Autodesk Inventor part; units mm, degrees
sketch "Sketch_2" plane through (0, 0, 0) normal (0, 1, 0) x (-1, 0, 0)
  line L0 (14.6744, 3.8205) -> (14.6744, 4.3333)
  line L1 (14.6744, 4.3333) -> (13.0333, 4.3333)
  arc A0 (13.0333, 4.3333) -> (12.1103, 3.4103) centre (13.0333, 3.4103) ccw
  line L2 (12.1103, 3.4103) -> (12.1103, 1.4103)
  arc A1 (11.7, 1) -> (12.1103, 1.4103) centre (11.7, 1.4103) ccw
  line L3 (11.7, 1) -> (-0.3, 1)
  arc A2 (-0.7103, 1.4103) -> (-0.3, 1) centre (-0.3, 1.4103) ccw
  line L4 (-0.7103, 1.4103) -> (-0.7103, 3.4103)
  arc A3 (-0.7103, 3.4103) -> (-1.6333, 4.3333) centre (-1.6333, 3.4103) ccw
  line L5 (-1.6333, 4.3333) -> (-3.2744, 4.3333)
  line L6 (-3.2744, 4.3333) -> (-3.2744, 3.8205)
  line L7 (-3.2744, 3.8205) -> (-1.6333, 3.8205)
  arc A4 (-1.2231, 3.4103) -> (-1.6333, 3.8205) centre (-1.6333, 3.4103) ccw
  line L8 (-1.2231, 3.4103) -> (-1.2231, 1.4103)
  arc A5 (-1.2231, 1.4103) -> (-0.3, 0.4872) centre (-0.3, 1.4103) ccw
  line L9 (-0.3, 0.4872) -> (11.7, 0.4872)
  arc A6 (11.7, 0.4872) -> (12.6231, 1.4103) centre (11.7, 1.4103) ccw
  line L10 (12.6231, 1.4103) -> (12.6231, 3.4103)
  arc A7 (13.0333, 3.8205) -> (12.6231, 3.4103) centre (13.0333, 3.4103) ccw
  line L11 (13.0333, 3.8205) -> (14.6744, 3.8205)
  dimension "d13" = 12
extrude "Extrusion1" add sketch "Sketch_2" along normal blind 161
sketch "Sketch_6" plane through (0, 0, 0) normal (0, 0, 1) x (1, 0, 0)
  arc A0 (-8.7098, 4.8974) -> (-3.5098, 4.8974) centre (-6.1098, 4.8974) ccw
  line L0 (-3.5098, 4.8974) -> (-3.5098, 17.6974)
  arc A1 (-3.5098, 17.6974) -> (-8.7098, 17.6974) centre (-6.1098, 17.6974) ccw
  line L1 (-8.7098, 17.6974) -> (-8.7098, 4.8974)
extrude "Extrusion2" cut sketch "Sketch_6" along normal blind 1
pattern_linear "Rectangular Pattern1" count 80 spacing 23 along (0, 1, 0) of "Extrusion2"
properties part number "PP0735H(1)"
Source: CAD feature listing. Evaluate the final solid. Frame: model axes, mm. A direction names the side the tool comes from. Round coordinates to 2 decimals unless told otherwise and drop trailing zeros. Write each loop counter-clockwise with the first axis right and the second up, starting at its lowest first coordinate (ties: lowest second). Pieces come first, ordered by that corner, then holes. Notation, with made-up numbers: M -10,-21 L 16,-21 A22 cw 16,-10 Z; hole C 46.5,63.25 d3. An arc over 180 degrees is marked long. Use CSV: the item, a comma, the result in double quotes. Start each with the question number.
Q1. Cut plane A-A on z = 2.2. Output: boundary loops of the cut face in (x, y).
Q2. First-contact query: P1, Ø0.6, axis at y = 99.5, z = 3, coming from the +X side; P2, Ø0.6, axis at y = 125.5, z = 0.5, coming from the +X side; P3, Ø1.5, axis at y = 77, z = 1.5, coming from the -X side. Flat tips, straight axial feed; report the tip coordinate or a pass-through.
Q3. Line query: line 1 (X direction, y = 121.5, z = 1.9); line 2 (Z direction, x = -1, y = 17); line 3 (X direction, y = 100, z = 0.85). Output: solid intervals per line, ascending. Write a range as from..to.
Q4. Pull-direction query (X, two-part tool) for faces 1 (the face through (-5.7, 161, 0.7)), 2 (the face through (-6.05, 48.3, 0.74)); classes: +X half, -X half, draft (parallel to the pull), parting line (faces both ways), or undercut.
Q5. Access query for faces 3 (the face through (-3, 79, 1)), 4 (the face through (-3, 79, 0.487)), 5 (the face through (-6.05, 71.3, 0.74)). Directions: +Z, -Z, +X, -X, +Y, -Y. A direction counts if a zero-diameter tool reaches every point of the face in a straight line with its end or side. Return the directions, or none.
Q6. Cut plane B-B on y = 23. Output: boundary loops of the cut face in (x, z).
Q7. Cut plane C-C on x = -6.5. Count the separate pieces of the cut face and the enclosed holes in it, plus the area to 3 significant figures.
Results found:
1,outline,"M -12.62,0 L -12.11,0 L -12.11,161 L -12.62,161 Z; M 0.71,0 L 1.22,0 L 1.22,161 L 0.71,161 Z"
2,P1,"x = 1.22"
2,P2,"x = 0.99"
2,P3,"x = -12.62"
3,line 1,"-12.62..-12.11, 0.71..1.22"
3,line 2,"0.49..1"
3,line 3,"-12.43..-8.71, -3.51..1.03"
4,face 1,"draft"
4,face 2,"undercut"
5,face 3,"+Z, +Y, -Y"
5,face 4,"-Z, +X, -X, +Y, -Y"
5,face 5,"+Z, -Z"
6,outline,"M -14.67,3.82 L -13.03,3.82 A0.41 cw -12.62,3.41 L -12.62,1.41 A0.92 ccw -11.7,0.49 L 0.3,0.49 A0.92 ccw 1.22,1.41 L 1.22,3.41 A0.41 cw 1.63,3.82 L 3.27,3.82 L 3.27,4.33 L 1.63,4.33 A0.92 ccw 0.71,3.41 L 0.71,1.41 A0.41 cw 0.3,1 L -11.7,1 A0.41 cw -12.11,1.41 L -12.11,3.41 A0.92 ccw -13.03,4.33 L -14.67,4.33 Z"
7,separate pieces,"8"
7,enclosed holes,"0"
7,area,"18.2 mm^2"
